Here's the drawing with two shaded views (mm, measured from the low corner). I have some questions. Give positions to 0.01 mm unless a question says otherwise; leave off trailing zeros. Write each loop counter-clockwise with the first axis right and the second up, starting at its lowest first coordinate (ties: lowest second). Pieces come first, ordered by that corner, then holes. Notation, with made-up numbers: M 20,-39.5 L 30,-39.5 A22 cw 30,-8.5 Z; hole C 21.25,72 d4. An arc over 180 degrees is marked long. Use one line per item in the form item = value. Start each with the question number.
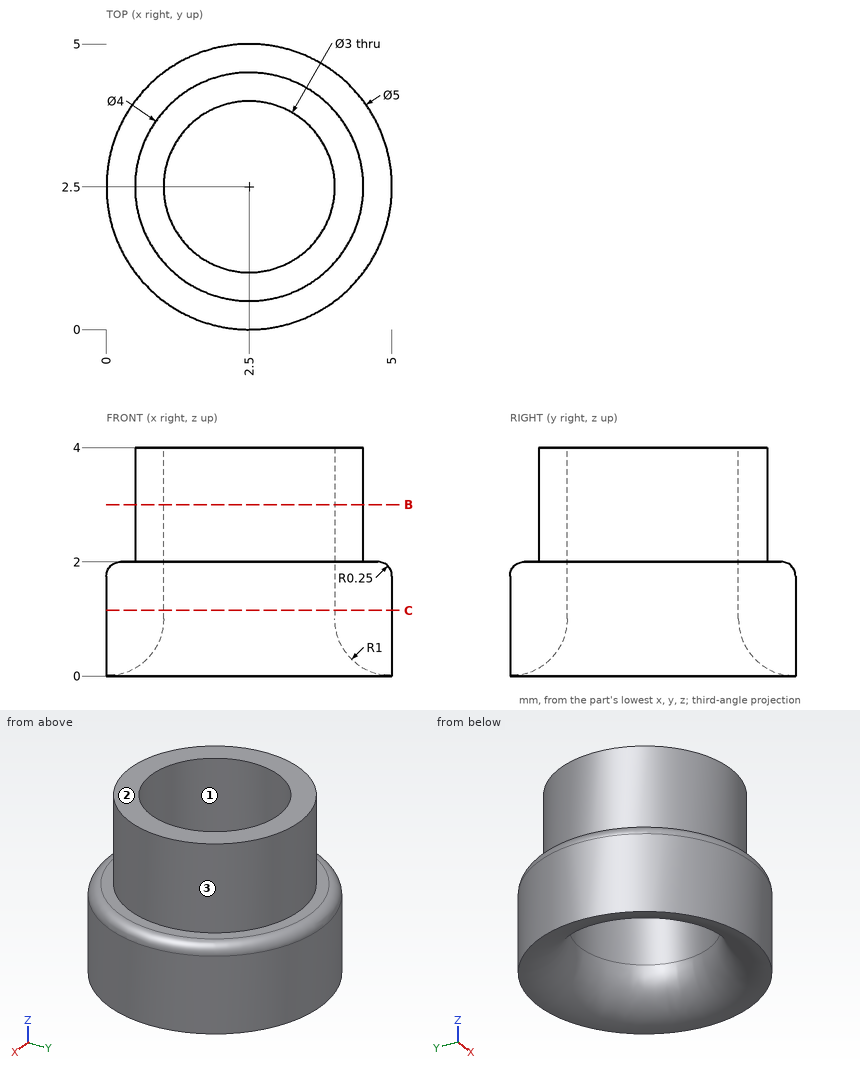
1) Please list where these lines run through material, in increasing order: line 1 (Y direction, x = 2.5, z = 1.65); line 2 (Y direction, x = 2.5, z = 3.45); line 3 (X direction, y = 1.5, z = 0.25) (1 decimal).
2) Will these pins go through, and if not, where does the flat tip stop? P1, Ø2, axis at x = 1, z = 1, coming from the -Y side; P2, Ø2, axis at y = 4, z = 1, coming from the +X side; P3, Ø2, axis at x = 3.5, y = 2.5, coming from the -Z side (1 decimal).
3) Thinking about a two-plate mould opening in Y: for the marked faces 1, 2 and 3, which applies, released by +Y, released by -Y, zero draft, split by the parting line, or undercut?
4) Suppose I cut it at B-B, the plane z = 3. List the corners of the cut face in (x, y) for me.
5) Suppose I cut it at C-C, the plane z = 1.15. List the corners of the cut face in (x, y) for me.
Checks:
q1.line_1 = 0 to 1, 4 to 5
q1.line_2 = 0.5 to 1, 4 to 4.5
q1.line_3 = 0.2 to 1, 4 to 4.8
q2.P1 = 0.05
q2.P2 = 4.95
q2.P3 = 0.1
q3.face_1 = undercut
q3.face_2 = zero draft
q3.face_3 = split by the parting line
q4.outline = C 2.5,2.5 d4; hole C 2.5,2.5 d3
q5.outline = C 2.5,2.5 d5; hole C 2.5,2.5 d3
